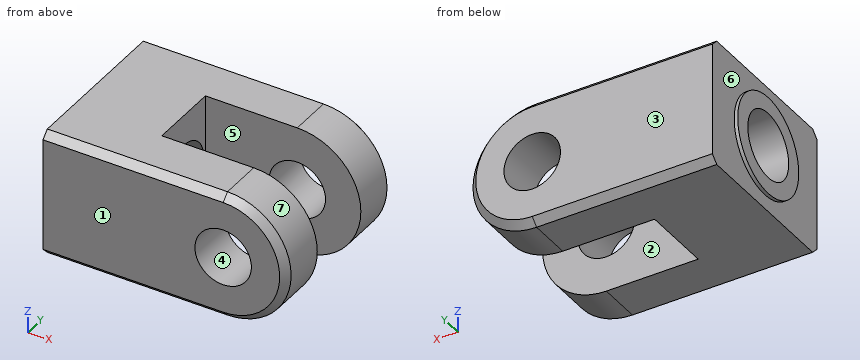
```python
from build123d import *

# Parameters (mm, degrees)
F0_R     = 12.7
F1_DEPTH = 38.1
F3_DEPTH = 38.1
F5_D     = 29.76626
F4_W     = 76.2
F4_H     = 57.15
F4_R     = 22.225
F6_DEPTH = 1.5875
F7_SIZE  = 3.175


with BuildPart() as f1:
    # F0 (on Front) → F1 (new body, symmetric)
    with BuildSketch(Plane.XZ):
        with BuildLine():
            Line((-55.5625, 28.575), (-55.5625, -28.575))
            Line((-55.5625, -28.575), (26.9875, -28.575))
            ThreePointArc((26.9875, -28.575), (55.5625, 0), (26.9875, 28.575))
            Line((26.9875, 28.575), (-55.5625, 28.575))
        make_face()
        with Locations((26.9875, 0)):
            Circle(F0_R, mode=Mode.SUBTRACT)
    extrude(amount=F1_DEPTH, both=True)

    # F2 (on Top) → F3 (cut, symmetric)
    with BuildSketch(Plane.XY):
        Polygon((55.5625, 0), (55.5625, 15.875), (-14.2875, 15.875), (-14.2875, 0), (-14.2875, -15.875), (55.5625, -15.875), align=None)
    extrude(amount=F3_DEPTH, both=True, mode=Mode.SUBTRACT)

    # F5 (through all)
    with Locations(Plane(origin=(-55.5625, 0, 0), x_dir=(0, -1, 0), z_dir=(-1, 0, 0))):
        with Locations((0, 0)):
            Hole(F5_D / 2)

    # F4 (on face) → F6 (cut)
    with BuildSketch(Plane(origin=(-55.5625, 0, 0), x_dir=(0, -1, 0), z_dir=(-1, 0, 0))):
        Rectangle(F4_W, F4_H)
        Circle(F4_R, mode=Mode.SUBTRACT)
    extrude(amount=-F6_DEPTH, mode=Mode.SUBTRACT)

    # F7
    f7_edges = [f1.edges().sort_by_distance(p)[0] for p in [
        (-13.49375, 38.1, 28.575),
        (-13.49375, -38.1, -28.575),
    ]]
    chamfer(f7_edges, length=F7_SIZE)


solid = f1.part
```
The listing builds one solid part. Answer for the finished solid, in the listing's coordinates (mm). Face numbers are marked on the shaded views. A direction names the side the tool comes from. Give positions to 0.01 mm unless a question says otherwise; leave off trailing zeros. Loops run counter-clockwise (first coordinate to the right, second up) from the corner with the lowest first, then second, coordinate; pieces in that order, holes last. Notation, with made-up numbers: M -3,-18 L 18,-18 A26 cw 18,12 Z; hole C 18,-21 d5. An arc over 180 degrees is marked long. One line per item, written item: value.
Q1. A cutting plane is placed at C-C on x = 4. Determine the outline of the cut face in (y, z) (3 decimals).
Working result:
outline: M -38.1,-25.4 L -34.925,-28.575 L -15.875,-28.575 L -15.875,28.575 L -34.925,28.575 L -38.1,25.4 Z; M 15.875,-28.575 L 34.925,-28.575 L 38.1,-25.4 L 38.1,25.4 L 34.925,28.575 L 15.875,28.575 Z
Q2. A cutting plane is placed at B-B on y = 0. Determine the outline of the cut face in (x, z) (1 decimal), then the cut area to 3 significant figures.
Working result:
outline: M -55.6,-22.2 L -54,-22.2 L -54,-28.6 L -14.3,-28.6 L -14.3,-14.9 L -55.6,-14.9 Z; M -55.6,14.9 L -14.3,14.9 L -14.3,28.6 L -54,28.6 L -54,22.2 L -55.6,22.2 Z
area: 1,110 mm^2
Q3. A cutting plane is placed at A-A on z = 0. Determine the outline of the cut face in (x, y) (1 decimal).
Working result:
outline: M -55.6,-22.2 L -54,-22.2 L -54,-38.1 L 14.3,-38.1 L 14.3,-15.9 L -14.3,-15.9 L -14.3,-14.9 L -55.6,-14.9 Z; M -55.6,14.9 L -14.3,14.9 L -14.3,15.9 L 14.3,15.9 L 14.3,38.1 L -54,38.1 L -54,22.2 L -55.6,22.2 Z; M 39.7,-38.1 L 52.4,-38.1 L 55.6,-34.9 L 55.6,-15.9 L 39.7,-15.9 Z; M 39.7,15.9 L 55.6,15.9 L 55.6,34.9 L 52.4,38.1 L 39.7,38.1 Z
Q4. For the marked faces 5, 6 and 7, determine the directions among +Z, -Z, +X, -X, +Y, -Y from which every point of the face is accessible in a straight line to the end or side of a thin tool.
Working result:
face 5: +Z, -Z, +X
face 6: -X
face 7: +X, +Y, -Y
Q5. Find the intervals of material crossed by line 1 (Z direction, x = 27, y = -34) (3 decimals); line 2 (Z direction, x = -44.5, y = 0) (3 decimals); line 3 (X direction, y = -26.5, z = 0) (1 decimal), in increasing order. Write a range as from..to.
Working result:
line 1: z = -28.575..-12.7, 12.7..28.575
line 2: z = -28.575..-14.883, 14.883..28.575
line 3: x = -54..14.3, 39.7..55.6
Q6. Flat-ended cylindrical pins translate along their axes: P1, Ø1.5, axis at y = 28, z = -1, coming from the -X side (3 decimals); P2, Ø2, axis at x = 41, y = 17, coming from the +Z side; P3, Ø20.5, axis at x = 26.99, z = 0, coming from the -Y side. Find the tip coordinate at first contact, or state that the pin passes through.
Working result:
P1: stops at x = -53.975
P2: stops at z = 25.44
P3: passes through
Q7. Determine the mould class of the marked faces 1, 2, 3 and 4 for opening direction Y: +Y half, -Y half, draft (parallel to the pull), parting line (faces both ways), or undercut.
Working result:
face 1: -Y half
face 2: undercut
face 3: +Y half
face 4: draft
